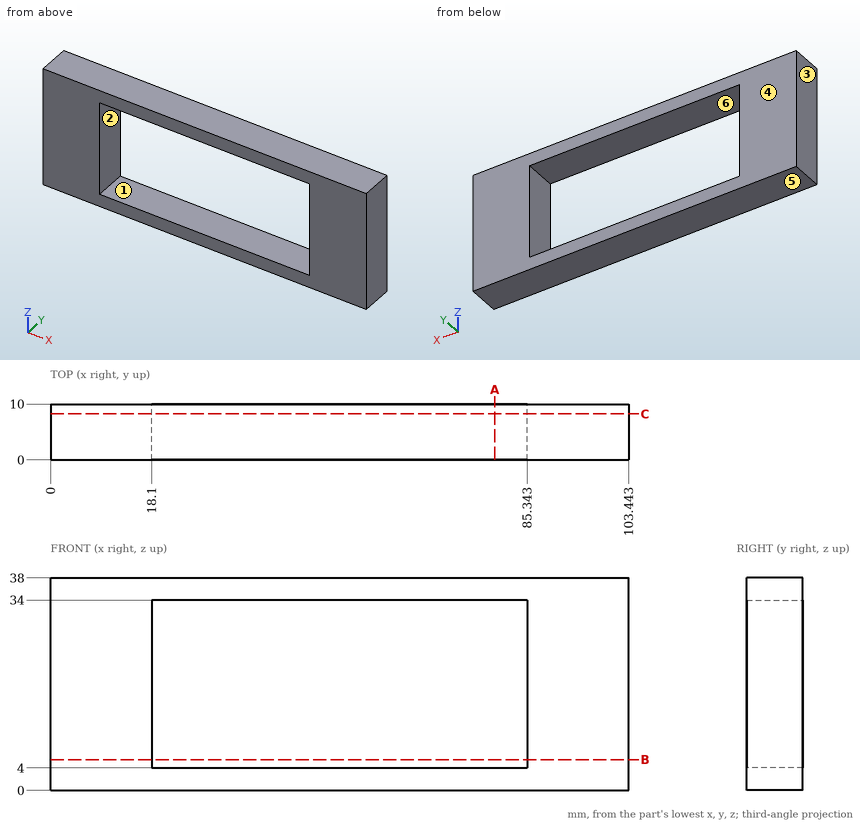
Design review of the part shown in the three views and the two pictorial views. Dimensions are in mm from the part's minimum x, y and z. A direction names the side the tool comes from. Give positions to 0.01 mm unless a question says otherwise; leave off trailing zeros. Write each loop counter-clockwise with the first axis right and the second up, starting at its lowest first coordinate (ties: lowest second). Pieces come first, ordered by that corner, then holes. Notation, with made-up numbers: M 63.25,89.5 L 74.25,89.5 A21 ccw 74.25,105.5 Z; hole C 32.25,1 d9. An arc over 180 degrees is marked long. One line per question, with ' | ' between items. Start each with the question number.
Item 1: We need section B-B on z = 5.5. Write out the cut boundary in (x, y).
Item 2: We need section A-A on x = 79.5. Write out the cut boundary in (y, z), plus the area to 3 significant figures.
Item 3: For pin 1 (1 mm diameter, centred on x = 20, z = 22.5, fed in from -Y), flat-tipped, find the tip position at first contact; note if it passes through.
Item 4: Wall thickness on line 1 (X direction, y = 2.5, z = 7); line 2 (Z direction, x = 53, y = 7.75): over which ranges is each line inside the solid? List them lowest first. Write a range as from..to.
Item 5: We need section C-C on y = 8.25. Write out the cut boundary in (x, z).
Item 6: Draft analysis for pull direction X (two halves, no side actions). For the marked faces 1, 2, 3 and 4, state which applies: released by +X, released by -X, zero draft, split by the parting line, or undercut.
Item 7: For the marked faces 5 and 6, list the 3-axis set-ups (+Z, -Z, +X, -X, +Y, -Y) from which the entire face can be reached by the end or side of a thin tool; tool diameter is ignored.
Results found:
1) outline: M 0,0 L 18.1,0 L 18.1,10 L 0,10 Z; M 85.34,0 L 103.44,0 L 103.44,10 L 85.34,10 Z
2) outline: M 0,0 L 10,0 L 10,4 L 0,4 Z; M 0,34 L 10,34 L 10,38 L 0,38 Z | area: 80.0 mm2
3) pin 1: passes through
4) line 1: x = 0..18.1, 85.34..103.44 | line 2: z = 0..4, 34..38
5) outline: M 0,0 L 103.44,0 L 103.44,38 L 0,38 Z; hole M 18.1,4 L 85.34,4 L 85.34,34 L 18.1,34 Z
6) face 1: undercut | face 2: undercut | face 3: released by -X | face 4: zero draft
7) face 5: -Z, +X, -X, +Y, -Y | face 6: +Y, -Y
